Part print with two shaded views. Sizes in mm from the minimum x, y, z corner. A direction names the side the tool comes from. Give positions to 0.01 mm unless a question says otherwise; leave off trailing zeros. Write each loop counter-clockwise with the first axis right and the second up, starting at its lowest first coordinate (ties: lowest second). Pieces come first, ordered by that corner, then holes. Notation, with made-up numbers: M 1.25,24 L 39.25,24 A26 cw 39.25,42 Z; hole C 13.25,-16 d8. An arc over 180 degrees is marked long. Return JSON: item names as keys, results as strings. Group by question number.
Q1. Wall check: probe 1 along Z at (x, y) = (12, 8); probe 2 along X at (y, z) = (12, 34.5); probe 3 along X at (y, z) = (23, 8.5). Give the ranges that are in metal, low to high.
Q2. Band-saw the part on C-C, the plane x = 9.5. Give the cut face in (y, z).
Q3. Band-saw the part on B-B, the plane z = 8. Give the cut face in (x, y).
Q4. Flat gauge pins, fed straight in: pin 1 Ø6 at (x, z) = (9, 28) entering from +Y; pin 2 Ø16 at (x, y) = (13, 27) entering from -Z; pin 3 Ø10 at (y, z) = (24.5, 21.5) entering from -X. Where does each tip first touch, or does it go through?
Q5. Band-saw the part on A-A, the plane y = 16.5. Give the cut face in (x, z), then the cut area to 3 significant figures.
Q6. Band-saw the part on D-D, the plane y = 34. Give the cut face in (x, z).
Q7. Tool access for the marked faces 1, 2 and 3: list every direction of +Z, -Z, +X, -X, +Y, -Y with a clear straight run to the whole face (end or side of a thin tool).
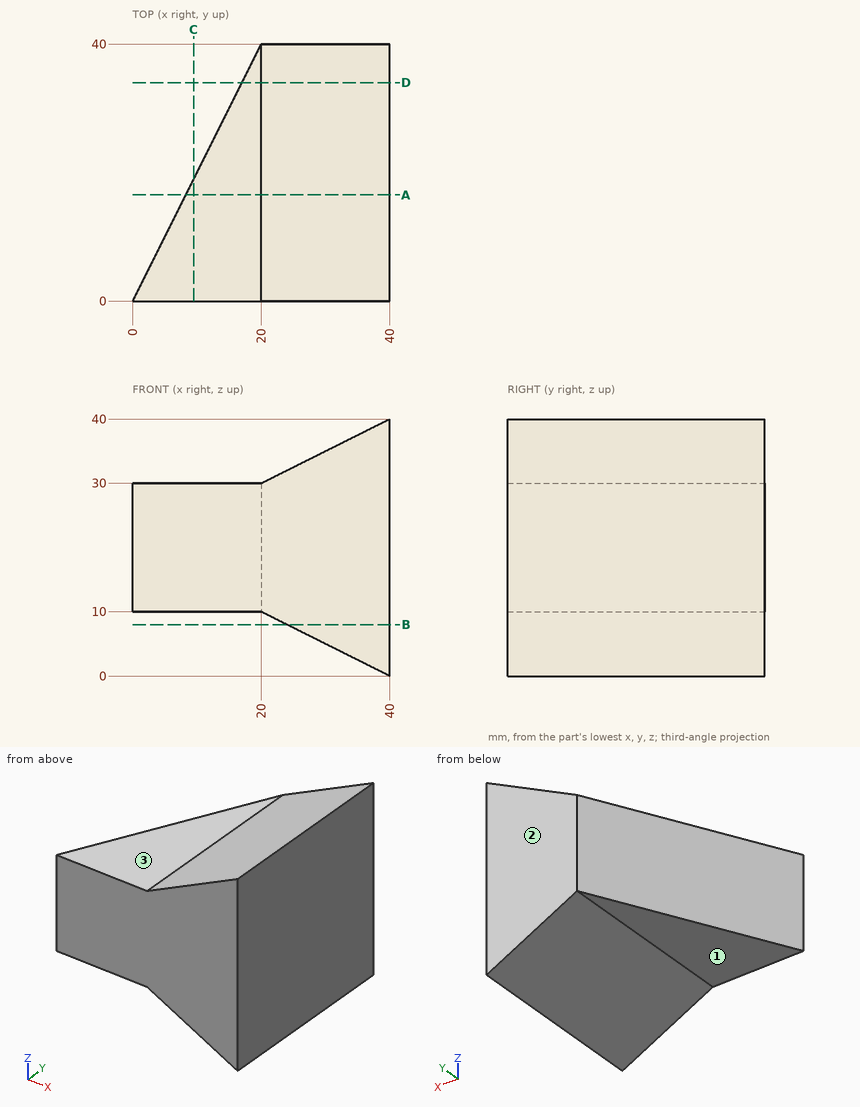
From the geometry:
{
 "1": {"probe 1": "z = 10 to 30", "probe 2": "x = 29 to 40", "probe 3": "x = 23 to 40"},
 "2": {"outline": "M 0,10 L 19,10 L 19,30 L 0,30 Z"},
 "3": {"outline": "M 24,0 L 40,0 L 40,40 L 24,40 Z"},
 "4": {"pin 1": "stops at y = 24", "pin 2": "stops at z = 9.5", "pin 3": "stops at x = 9.75"},
 "5": {"outline": "M 8.25,10 L 20,10 L 40,0 L 40,40 L 20,30 L 8.25,30 Z", "area": "835 mm^2"},
 "6": {"outline": "M 17,10 L 20,10 L 40,0 L 40,40 L 20,30 L 17,30 Z"},
 "7": {"face 1": "-Z, -X, +Y, -Y", "face 2": "+Z, -Z, +X, -X, +Y", "face 3": "+Z, -X, +Y, -Y"}
}
